CAD build for the part. Positions are in the model's coordinates, mm. Face numbers are marked on the shaded views. A direction names the side the tool comes from. Round coordinates to 2 decimals unless told otherwise and drop trailing zeros. Order: outer loops, then holes, each group sorted by start corner. A loop starts at its lowest first (then second) coordinate and runs counter-clockwise, first axis right, second up. Notation, with made-up numbers: (86.5, 36.5) - (112.5, 36.5) arc R24 cw to (112.5, 55.5) - close; hole circle Ø4 at (19.5, 12). An arc over 180 degrees is marked (long way). Write item = value, one per line.
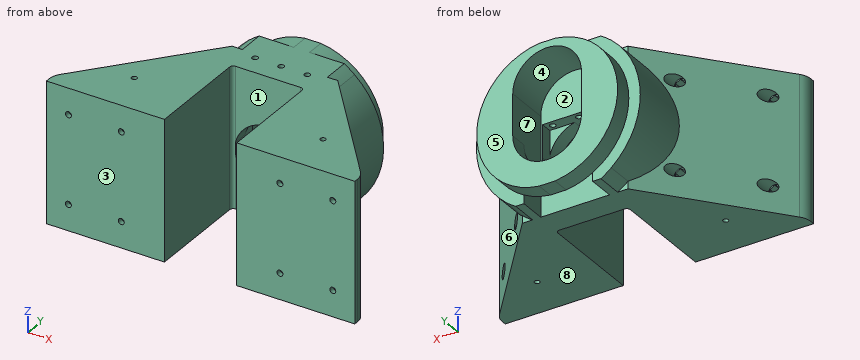
from build123d import *

# Parameters (mm, degrees)
BOSS_EXTRUDE2_START   = -32.75
BOSS_EXTRUDE2_DEPTH   = 79.5
CUT_EXTRUDE1_DEPTH    = 117.042459902
SKETCH6_R             = 1.7
CUT_EXTRUDE2_DEPTH    = 125.486354674
CUT_EXTRUDE3_START    = -3
CUT_EXTRUDE3_DEPTH    = 122.486354674
CUT_EXTRUDE8_START    = -15
SKETCH17_R            = 3.5
CUT_EXTRUDE8_DEPTH    = 110.486354674
CUT_EXTRUDE9_START    = -52
SKETCH18_R            = 3.5
CUT_EXTRUDE9_DEPTH    = 73.486354674
FILLET1_R             = 2
FILLET3_R             = 10
CUT_EXTRUDE5_REACH    = 142.113
SKETCH10_R            = 1.65
CUT_EXTRUDE6_REACH    = 142.113
SKETCH11_R            = 1.5
BOSS_EXTRUDE4_DEPTH   = 8.5
BOSS_EXTRUDE5_START   = -66.421548224
BOSS_EXTRUDE5_DEPTH   = 81.421548224
BOSS_EXTRUDE5_2_DEPTH = 15
BOSS_EXTRUDE6_DEPTH   = 10


with BuildPart() as part:
    # Sketch3 → Boss-Extrude2 (new body)
    with BuildSketch(Plane.XY.offset(BOSS_EXTRUDE2_START)):
        Polygon((-20.5, 0), (-87.5, 0), (-87.5, 6), (-30, 75.2), (0, 75.2), (0, 60.2), (-20.5, 60.2), align=None)
    boss_extrude2 = extrude(amount=BOSS_EXTRUDE2_DEPTH)

    # Mirror1: Boss-Extrude2 across plane
    add(boss_extrude2.mirror(Plane(origin=(0, 75.2, -32.75), x_dir=(0, 0, 1), z_dir=(1, 0, 0))))

    # Sketch4 → Cut-Extrude1 (cut, through all)
    with BuildSketch(Plane.XZ.offset(-60.2)):
        with BuildLine():
            Line((-18.5, 0), (-18.5, 18.5))
            Line((-18.5, 18.5), (18.5, 18.5))
            Line((18.5, 18.5), (18.5, 0))
            ThreePointArc((18.5, 0), (0, -18.5), (-18.5, 0))
        make_face()
    extrude(amount=-CUT_EXTRUDE1_DEPTH, mode=Mode.SUBTRACT)

    # Sketch6 → Cut-Extrude2 (cut, through all)
    with BuildSketch(Plane.XZ):
        with Locations((-75, 32)):
            Circle(SKETCH6_R)
        with Locations((-75, -18)):
            Circle(SKETCH6_R)
        with Locations((75, 32)):
            Circle(SKETCH6_R)
        with Locations((75, -18)):
            Circle(SKETCH6_R)
        with Locations((-45, 32)):
            Circle(SKETCH6_R)
        with Locations((-45, -18)):
            Circle(SKETCH6_R)
        with Locations((45, 32)):
            Circle(SKETCH6_R)
        with Locations((45, -18)):
            Circle(SKETCH6_R)
    extrude(amount=-CUT_EXTRUDE2_DEPTH, mode=Mode.SUBTRACT)

    # Sketch7 → Cut-Extrude3 (cut, through all)
    with BuildSketch(Plane.XZ.offset(CUT_EXTRUDE3_START)):
        Polygon((-75, 35.175426481), (-77.75, 33.58771324), (-77.75, 30.41228676), (-75, 28.824573519), (-72.25, 30.41228676), (-72.25, 33.58771324), align=None)
        Polygon((-75, -14.824573519), (-77.75, -16.41228676), (-77.75, -19.58771324), (-75, -21.175426481), (-72.25, -19.58771324), (-72.25, -16.41228676), align=None)
        Polygon((-45, -14.824573519), (-47.75, -16.41228676), (-47.75, -19.58771324), (-45, -21.175426481), (-42.25, -19.58771324), (-42.25, -16.41228676), align=None)
        Polygon((-45, 35.175426481), (-47.75, 33.58771324), (-47.75, 30.41228676), (-45, 28.824573519), (-42.25, 30.41228676), (-42.25, 33.58771324), align=None)
        Polygon((45, -14.824573519), (42.25, -16.41228676), (42.25, -19.58771324), (45, -21.175426481), (47.75, -19.58771324), (47.75, -16.41228676), align=None)
        Polygon((75, -14.824573519), (72.25, -16.41228676), (72.25, -19.58771324), (75, -21.175426481), (77.75, -19.58771324), (77.75, -16.41228676), align=None)
        Polygon((75, 35.175426481), (72.25, 33.58771324), (72.25, 30.41228676), (75, 28.824573519), (77.75, 30.41228676), (77.75, 33.58771324), align=None)
        Polygon((45, 35.175426481), (42.25, 33.58771324), (42.25, 30.41228676), (45, 28.824573519), (47.75, 30.41228676), (47.75, 33.58771324), align=None)
    extrude(amount=-CUT_EXTRUDE3_DEPTH, mode=Mode.SUBTRACT)

    # Sketch17 → Cut-Extrude8 (cut, through all)
    with BuildSketch(Plane.XZ.offset(CUT_EXTRUDE8_START)):
        with Locations((-75, 32)):
            Circle(SKETCH17_R)
        with Locations((-75, -18)):
            Circle(SKETCH17_R)
        with Locations((75, 32)):
            Circle(SKETCH17_R)
        with Locations((75, -18)):
            Circle(SKETCH17_R)
    extrude(amount=-CUT_EXTRUDE8_DEPTH, mode=Mode.SUBTRACT)

    # Sketch18 → Cut-Extrude9 (cut, through all)
    with BuildSketch(Plane.XZ.offset(CUT_EXTRUDE9_START)):
        with Locations((-45, 32)):
            Circle(SKETCH18_R)
        with Locations((-45, -18)):
            Circle(SKETCH18_R)
        with Locations((45, -18)):
            Circle(SKETCH18_R)
        with Locations((45, 32)):
            Circle(SKETCH18_R)
    extrude(amount=-CUT_EXTRUDE9_DEPTH, mode=Mode.SUBTRACT)

    # Fillet1
    fillet1_edges = [part.edges().sort_by_distance(p)[0] for p in [
        (-20.5, 60.2, 7),
        (20.5, 60.2, 7),
    ]]
    fillet(fillet1_edges, radius=FILLET1_R - 0.0001)  # a hair under: the kernel refuses the full size

    # Fillet3
    fillet3_edges = [part.edges().sort_by_distance(p)[0] for p in [
        (-87.5, 6, 7),
        (87.5, 6, 7),
    ]]
    fillet(fillet3_edges, radius=FILLET3_R)

    # Sketch10 → Cut-Extrude5 (cut, up to next)
    with BuildSketch(Plane.XY.offset(46.75), mode=Mode.PRIVATE) as cut_extrude5_sk1:
        with Locations((0, 71.9)):
            Circle(SKETCH10_R)
    cut_extrude5_tool1 = extrude(cut_extrude5_sk1.sketch, amount=-CUT_EXTRUDE5_REACH, mode=Mode.PRIVATE) & part.part
    # Sketch10 → Cut-Extrude5 (cut, up to next)
    with BuildSketch(Plane.XY.offset(46.75), mode=Mode.PRIVATE) as cut_extrude5_sk2:
        with Locations((-14.8, 71.9)):
            Circle(SKETCH10_R)
    cut_extrude5_tool2 = extrude(cut_extrude5_sk2.sketch, amount=-CUT_EXTRUDE5_REACH, mode=Mode.PRIVATE) & part.part
    # Sketch10 → Cut-Extrude5 (cut, up to next)
    with BuildSketch(Plane.XY.offset(46.75), mode=Mode.PRIVATE) as cut_extrude5_sk3:
        with Locations((14.8, 71.9)):
            Circle(SKETCH10_R)
    cut_extrude5_tool3 = extrude(cut_extrude5_sk3.sketch, amount=-CUT_EXTRUDE5_REACH, mode=Mode.PRIVATE) & part.part
    add(cut_extrude5_tool1.solids().sort_by_distance((0, 71.9, 46.75))[0], mode=Mode.SUBTRACT)
    add(cut_extrude5_tool2.solids().sort_by_distance((-14.8, 71.9, 46.75))[0], mode=Mode.SUBTRACT)
    add(cut_extrude5_tool3.solids().sort_by_distance((14.8, 71.9, 46.75))[0], mode=Mode.SUBTRACT)

    # Sketch11 → Cut-Extrude6 (cut, up to next)
    with BuildSketch(Plane.XY.offset(46.75), mode=Mode.PRIVATE) as cut_extrude6_sk1:
        with Locations((-53.5, 25)):
            Circle(SKETCH11_R)
    cut_extrude6_tool1 = extrude(cut_extrude6_sk1.sketch, amount=-CUT_EXTRUDE6_REACH, mode=Mode.PRIVATE) & part.part
    # Sketch11 → Cut-Extrude6 (cut, up to next)
    with BuildSketch(Plane.XY.offset(46.75), mode=Mode.PRIVATE) as cut_extrude6_sk2:
        with Locations((53.5, 25)):
            Circle(SKETCH11_R)
    cut_extrude6_tool2 = extrude(cut_extrude6_sk2.sketch, amount=-CUT_EXTRUDE6_REACH, mode=Mode.PRIVATE) & part.part
    add(cut_extrude6_tool1.solids().sort_by_distance((-53.5, 25, 46.75))[0], mode=Mode.SUBTRACT)
    add(cut_extrude6_tool2.solids().sort_by_distance((53.5, 25, 46.75))[0], mode=Mode.SUBTRACT)

    # Sketch13 → Boss-Extrude4 (add)
    with BuildSketch(Plane.XZ.offset(-60.2)):
        with BuildLine():
            Line((-18.5, 18.5), (-18.5, 4.330127019))
            ThreePointArc((-18.5, 4.330127019), (-13.435028843, 13.435028843), (-4.330127019, 18.5))
            Line((-4.330127019, 18.5), (-18.5, 18.5))
        make_face()
        with BuildLine():
            Line((18.5, 18.5), (4.330127019, 18.5))
            ThreePointArc((4.330127019, 18.5), (13.435028843, 13.435028843), (18.5, 4.330127019))
            Line((18.5, 4.330127019), (18.5, 18.5))
        make_face()
    extrude(amount=-BOSS_EXTRUDE4_DEPTH)

    # Boss-Extrude5: read off the stored shape, not the designer's step
    # Boss-Extrude5 outline → Boss-Extrude5 (add)
    with BuildSketch(Plane(origin=(0, 75.2, 0), x_dir=(1, 0, 0), z_dir=(0, 1, 0)).offset(BOSS_EXTRUDE5_START)):
        with BuildLine():
            Line((-30, -42.528157847), (-30, 28.528157847))
            ThreePointArc((-30, 28.528157847), (-46.5, -7), (-30, -42.528157847))
        make_face()
        with BuildLine():
            ThreePointArc((30, -42.528157847), (46.5, -7), (30, 28.528157847))
            Line((30, 28.528157847), (30, -42.528157847))
        make_face()
    extrude(amount=BOSS_EXTRUDE5_DEPTH)

    # Boss-Extrude5 2 outline → Boss-Extrude5 2 (add)
    with BuildSketch(Plane(origin=(0, 75.2, 0), x_dir=(1, 0, 0), z_dir=(0, 1, 0))):
        with BuildLine():
            Line((-19.5, 32.75), (-24.128561913, 32.75))
            ThreePointArc((-24.128561913, 32.75), (-27.146478436, 30.753393338), (-30, 28.528157847))
            Line((-30, 28.528157847), (-30, -42.528157847))
            ThreePointArc((-30, -42.528157847), (-27.146478436, -44.753393338), (-24.128561913, -46.75))
            Line((-24.128561913, -46.75), (24.128561913, -46.75))
            ThreePointArc((24.128561913, -46.75), (27.146478436, -44.753393338), (30, -42.528157847))
            Line((30, -42.528157847), (30, 28.528157847))
            ThreePointArc((30, 28.528157847), (27.146478436, 30.753393338), (24.128561913, 32.75))
            Line((24.128561913, 32.75), (19.5, 32.75))
            Line((19.5, 32.75), (19.5, -23.5))
            ThreePointArc((19.5, -23.5), (0, -43), (-19.5, -23.5))
            Line((-19.5, -23.5), (-19.5, 32.75))
        make_face()
    extrude(amount=BOSS_EXTRUDE5_2_DEPTH)

    # Sketch15 → Boss-Extrude6 (add)
    with BuildSketch(Plane(origin=(0, 90.2, 0), x_dir=(1, 0, 0), z_dir=(0, 1, 0))):
        with BuildLine():
            Line((-4.465142775, 32.75), (4.465142775, 32.75))
            ThreePointArc((4.465142775, 32.75), (40, -7), (4.465142775, -46.75))
            Line((4.465142775, -46.75), (-4.465142775, -46.75))
            ThreePointArc((-4.465142775, -46.75), (-40, -7), (-4.465142775, 32.75))
        make_face()
        with BuildLine():
            Line((19.5, -23.5), (19.5, 0))
            ThreePointArc((19.5, 0), (0, 19.5), (-19.5, 0))
            Line((-19.5, 0), (-19.5, -23.5))
            ThreePointArc((-19.5, -23.5), (0, -43), (19.5, -23.5))
        make_face(mode=Mode.SUBTRACT)
    extrude(amount=BOSS_EXTRUDE6_DEPTH)


solid = part.part
(1) Band-saw the part on A-A on z = 14.5. Count the separate pieces of the cut face and the enclosed holes in it, plus the area to 3 significant figures.
Solved:
separate_pieces = 2
enclosed_holes = 2
area = 7,740 mm²
(2) Probe line 1 along X through (y, z) = (23.25, 32); line 2 along Y through (x, z) = (-14.8, 26.5); line 3 along Z through (x, y) = (-75, 17.75). List the from-to ranges inside material, lowest first.
Solved:
line_1 = -71.5 to -47.75, -42.25 to -20.5, 20.5 to 42.25, 47.75 to 71.5
line_2 = 60.2 to 70.25, 73.55 to 75.2
line_3 = -32.75 to -21.5, -14.5 to 28.5, 35.5 to 46.75
(3) Band-saw the part on B-B on y = 93. List the corners of the cut face in (x, z), plus the area to 3 significant figures.
Solved:
outline = (-4.47, -32.75) - (4.47, -32.75) arc R40 ccw to (4.47, 46.75) - (-4.47, 46.75) arc R40 ccw to start; hole (-19.5, 0) arc R19.5 ccw to (19.5, 0) - (19.5, 23.5) arc R19.5 ccw to (-19.5, 23.5) - close
area = 2,910 mm²
(4) Tool access for the marked faces 1, 2, 3, 4 and 5: list every direction of +Z, -Z, +X, -X, +Y, -Y with a clear straight run to the whole face (end or side of a thin tool).
Solved:
face_1 = +Z, -Z, -Y
face_2 = -Z
face_3 = +Z, -Z, +X, -X, -Y
face_4 = +Y
face_5 = +Z, -Z, +X, -X, +Y
(5) Band-saw the part on D-D on x = -32. List the corners of the cut face in (y, z), plus the area to 3 significant figures.
Solved:
outline = (0, -32.75) - (72.79, -32.75) - (72.79, -26.74) - (90.2, -26.74) - (90.2, -17) - (100.2, -17) - (100.2, 31) - (90.2, 31) - (90.2, 40.74) - (72.79, 40.74) - (72.79, 46.75) - (0, 46.75) - close
area = 7,440 mm²
(6) Pull direction Z, two halves, no side cores. Call the marked faces 6, 7 and 8: released by +Z, released by -Z, zero draft, split by the parting line, or undercut.
Solved:
face_6 = zero draft
face_7 = undercut
face_8 = released by -Z
(7) Band-saw the part on C-C on x = 10. List the corners of the cut face in (y, z).
Solved:
outline = (60.2, -32.75) - (75.2, -32.75) - (75.2, -15.56) - (60.2, -15.56) - close; (60.2, 16.16) - (68.7, 16.16) - (68.7, 18.5) - (75.2, 18.5) - (75.2, 40.24) - (100.2, 40.24) - (100.2, 45.73) - (90.2, 45.73) - (90.2, 46.75) - (60.2, 46.75) - close; (90.2, -31.73) - (100.2, -31.73) - (100.2, -16.74) - (90.2, -16.74) - close
(8) Drop flat-ended pins along their axis: pin 1 (1.6 mm diameter, centred on x = -45, z = 30.5, fed in from +Y); pin 2 (8 mm diameter, centred on x = 62, y = 43, fed in from +Z); pin 3 (3.5 mm diameter, centred on x = 27.5, z = 45, fed in from +Y); pin 4 (2.5 mm diameter, centred on y = 28.5, z = 32.5, fed in from +X). Give the stop position or say it passes through.
Solved:
pin_1 = 3
pin_2 = through
pin_3 = 90.2
pin_4 = 69.84
